Design review of the part built by this model. Coordinates are the model's own, in mm. A direction names the side the tool comes from. Round coordinates to 2 decimals unless told otherwise and drop trailing zeros. Loops run counter-clockwise (first coordinate to the right, second up) from the corner with the lowest first, then second, coordinate; pieces in that order, holes last. Notation, with made-up numbers: (15.25, -32.75) - (58.25, -32.75) arc R18 ccw to (58.25, -23.75) - close; hole circle Ø10 at (66.25, -38.75). An arc over 180 degrees is marked (long way). Return JSON: item names as keys, results as strings. Group by question number.
from build123d import *

# Parameters (mm, degrees)
SKETCH1_W           = 70
SKETCH1_H           = 85
BOSS_EXTRUDE1_DEPTH = 25
SKETCH2_W           = 18
SKETCH2_H           = 75
CUT_EXTRUDE1_DEPTH  = 10


with BuildPart() as part:
    # Sketch1 → Boss-Extrude1 (new body)
    with BuildSketch(Plane(origin=(0, 0, 0), x_dir=(1, 0, 0), z_dir=(0, 1, 0))):
        Rectangle(SKETCH1_W, SKETCH1_H)
    extrude(amount=BOSS_EXTRUDE1_DEPTH)

    # Sketch2 → Cut-Extrude1 (cut)
    with BuildSketch(Plane(origin=(0, 25, 0), x_dir=(1, 0, 0), z_dir=(0, 1, 0))):
        with Locations((-21, 0)):
            Rectangle(SKETCH2_W, SKETCH2_H)
        Rectangle(SKETCH2_W, SKETCH2_H)
        with Locations((21, 0)):
            Rectangle(SKETCH2_W, SKETCH2_H)
    extrude(amount=-CUT_EXTRUDE1_DEPTH, mode=Mode.SUBTRACT)


solid = part.part
Q1. Draft analysis for pull direction X (two halves, no side actions). For faces 1 (the flat face through (30, 20, 1)), 2 (the flat face through (35, 12, 1)), 3 (the flat face through (-11, 25, 6)), state which applies: pulls with the +X half, pulls with the -X half, needs draft (parallel to the pull), parting line crosses it, or undercut.
Q2. Add section B-B, the plane x = 15. State the section outline as (y, z) points, plus the area to 4 significant figures.
Q3. For line 1 (X direction, y = 24, z = -30.5); line 2 (Z direction, x = -1, y = 16.25); line 3 (Y direction, x = 29, z = -30), list the stretches that pass through material, from the lowest coordinate up.
Q4. Add section A-A, the plane y = 20.75. State the section outline as (x, z) points.
Q5. Insertion check: pin 1 Ø20 at (x, z) = (3.5, 2.5) entering from +Y; pin 2 Ø4 at (x, z) = (6.5, 31) entering from +Y. Each pin has a flat end and moves straight along its axis. Give the tip position at first contact, or say it passes through.
Q6. Add section C-C, the plane z = -19.5. State the section outline as (x, y) points.
Q7. Tool access review of faces 4 (the flat face through (0, 15, -1)), 5 (the flat face through (0, 12, -42.5)): name each direction out of +Z, -Z, +X, -X, +Y, -Y from which nothing blocks a thin tool from reaching the whole face with its end or side.
Evaluation:
{
 "1": {"face 1": "undercut", "face 2": "pulls with the +X half", "face 3": "needs draft"},
 "2": {"outline": "(0, -42.5) - (25, -42.5) - (25, -37.5) - (15, -37.5) - (15, 37.5) - (25, 37.5) - (25, 42.5) - (0, 42.5) - close", "area": "1,375 mm²"},
 "3": {"line 1": "-35 to -30, -12 to -9, 9 to 12, 30 to 35", "line 2": "-42.5 to -37.5, 37.5 to 42.5", "line 3": "0 to 15"},
 "4": {"outline": "(-35, -42.5) - (35, -42.5) - (35, 42.5) - (-35, 42.5) - close; hole (-30, -37.5) - (-12, -37.5) - (-12, 37.5) - (-30, 37.5) - close; hole (-9, -37.5) - (9, -37.5) - (9, 37.5) - (-9, 37.5) - close; hole (12, -37.5) - (30, -37.5) - (30, 37.5) - (12, 37.5) - close"},
 "5": {"pin 1": "y = 25", "pin 2": "y = 15"},
 "6": {"outline": "(-35, 0) - (35, 0) - (35, 25) - (30, 25) - (30, 15) - (12, 15) - (12, 25) - (9, 25) - (9, 15) - (-9, 15) - (-9, 25) - (-12, 25) - (-12, 15) - (-30, 15) - (-30, 25) - (-35, 25) - close"},
 "7": {"face 4": "+Y", "face 5": "-Z, +X, -X, +Y, -Y"}
}
